```python
from build123d import *

# Parameters (mm, degrees)
BOSS_EXTRUDE1_DEPTH             = 1.5
BOSS_EXTRUDE2_DEPTH             = 1.5
BOSS_EXTRUDE3_DEPTH             = 1.5
CUT_EXTRUDE1_START              = -4
SKETCH2_R                       = 2.25
CUT_EXTRUDE1_DEPTH              = 5
CIRPATTERN1_COUNT               = 3
CIRPATTERN1_ANGLE               = 60
CIRPATTERN1_THE_OTHER_WAY_COUNT = 3
CIRPATTERN1_THE_OTHER_WAY_ANGLE = 60
CUT_EXTRUDE2_START              = -4
SKETCH6_R                       = 3.25
CUT_EXTRUDE2_DEPTH              = 5
LPATTERN1_COUNT                 = 3
LPATTERN1_PITCH                 = 12.5
SKETCH7_R                       = 3.25
CUT_EXTRUDE3_DEPTH              = 10
LPATTERN2_COUNT                 = 4
LPATTERN2_PITCH                 = 12


with BuildPart() as part:
    # Sketch1 → Boss-Extrude1 (new body, symmetric)
    with BuildSketch(Plane(origin=(0, 0, 0), x_dir=(1, 0, 0), z_dir=(0, 1, 0))):
        with BuildLine():
            Line((0, 33), (0, 43))
            ThreePointArc((0, 43), (41.53481053, 11.129218939), (21.5, -37.239092363))
            Line((21.5, -37.239092363), (16.5, -28.578838325))
            ThreePointArc((16.5, -28.578838325), (31.875552268, 8.541028488), (0, 33))
        make_face()
    extrude(amount=BOSS_EXTRUDE1_DEPTH, both=True)

    # Sketch4 → Boss-Extrude2 (add, symmetric)
    with BuildSketch(Plane(origin=(0, 0, 0), x_dir=(1, 0, 0), z_dir=(0, 1, 0))):
        Polygon((90.122106501, 50.030050167), (25.40507614, 32.689174146), (38.346028395, -15.607117169), (103.063058756, 1.733758853), align=None)
    extrude(amount=BOSS_EXTRUDE2_DEPTH, both=True)

    # Sketch5 → Boss-Extrude3 (add, symmetric)
    with BuildSketch(Plane(origin=(0, 0, 0), x_dir=(1, 0, 0), z_dir=(0, 1, 0))):
        Polygon((0, 43), (58.722616268, 41.616582117), (27.323126035, 33.203114066), align=None)
        Polygon((71.663568523, -6.679709198), (40.26407829, -15.093177248), (21.5, -37.239092363), align=None)
    extrude(amount=BOSS_EXTRUDE3_DEPTH, both=True)

    # Sketch2 → Cut-Extrude1 (cut)
    with BuildSketch(Plane(origin=(0, 1.5, 0), x_dir=(1, 0, 0), z_dir=(0, 1, 0)).offset(CUT_EXTRUDE1_START)):
        with Locations((36.757261811, 9.638656763)):
            Circle(SKETCH2_R)
    cut_extrude1 = extrude(amount=CUT_EXTRUDE1_DEPTH, mode=Mode.SUBTRACT)

    # CirPattern1: Cut-Extrude1 ×3 about axis
    cirpattern1_axis = Axis((0, 0, 0), (0, -1, 0))
    for i in range(1, CIRPATTERN1_COUNT):
        add(cut_extrude1.rotate(cirpattern1_axis, i * CIRPATTERN1_ANGLE / (CIRPATTERN1_COUNT - 1)), mode=Mode.SUBTRACT)

    # CirPattern1 the other way: Cut-Extrude1 ×3 about axis
    cirpattern1_the_other_way_axis = Axis((0, 0, 0), (0, 1, 0))
    for i in range(1, CIRPATTERN1_THE_OTHER_WAY_COUNT):
        add(cut_extrude1.rotate(cirpattern1_the_other_way_axis, i * CIRPATTERN1_THE_OTHER_WAY_ANGLE / (CIRPATTERN1_THE_OTHER_WAY_COUNT - 1)), mode=Mode.SUBTRACT)

    # Sketch6 → Cut-Extrude2 (cut)
    with BuildSketch(Plane(origin=(0, 1.5, 0), x_dir=(1, 0, 0), z_dir=(0, 1, 0)).offset(CUT_EXTRUDE2_START)):
        with Locations((94.679313348, 9.840102845)):
            Circle(SKETCH6_R)
        with Locations((86.914741995, 38.817877634)):
            Circle(SKETCH6_R)
    cut_extrude2 = extrude(amount=CUT_EXTRUDE2_DEPTH, mode=Mode.SUBTRACT)

    # LPattern1: Cut-Extrude2 ×3
    with Locations(*[Vector(-0.965925826, 0, 0.258819045) * (i * LPATTERN1_PITCH) for i in range(1, LPATTERN1_COUNT)]):
        add(cut_extrude2, mode=Mode.SUBTRACT)

    # Sketch7 → Cut-Extrude3 (cut)
    with BuildSketch(Plane(origin=(0, 1.5, 0), x_dir=(1, 0, 0), z_dir=(0, 1, 0))):
        with Locations((90.797027671, 24.32899024)):
            Circle(SKETCH7_R)
    cut_extrude3 = extrude(amount=-CUT_EXTRUDE3_DEPTH, mode=Mode.SUBTRACT)

    # LPattern2: Cut-Extrude3 ×4
    with Locations(*[Vector(-0.965925826, 0, 0.258819045) * (i * LPATTERN2_PITCH) for i in range(1, LPATTERN2_COUNT)]):
        add(cut_extrude3, mode=Mode.SUBTRACT)


solid = part.part
```
CAD build for the part. Positions are in the model's coordinates, mm. Give positions to 0.01 mm unless a question says otherwise; leave off trailing zeros. Write each loop counter-clockwise with the first axis right and the second up, starting at its lowest first coordinate (ties: lowest second). Pieces come first, ordered by that corner, then holes. Notation, with made-up numbers: M 12.5,17.25 L 16.5,17.25 A32 ccw 16.5,47.25 Z; hole C 8,80 d11. An arc over 180 degrees is marked long. Return JSON: item names as keys, results as strings. Group by question number.
(1) Drill centre lines: L1, parallel to Z at x = 36, y = 1.1; L2, parallel to Z at x = 38, y = 0.4; L3, parallel to X at y = 1.2, z = -22.5. Where is each one in solid material? Low to high. Write a range as [from, to].
(2) Band-saw the part on A-A (x = 31.5). Give the cut face in (y, z), and give its area (3 significant figures).
(3) Flat gauge pin, fed straight in: pin 1 Ø1 at (x, y) = (40, 1) entering from -Z. Where does the tip first touch, or does it go through?
(4) Band-saw the part on B-B (y = 0.65). State how many separate pieces and enclosed holes the cut face has, and give its area (3 significant figures).
(5) Band-saw the part on D-D (z = 20.5). Give the cut face in (x, y), and give its area (3 significant figures).
(6) Band-saw the part on C-C (x = 61). Give the cut face in (y, z).
(7) Mould opens along X. For faces 1 (the face through (28.384, -0.021, 28.534)), 2 (the face through (51, -1.5, -17)), 3 (the face through (96.683, 0.021, -25.544)) say: pulls with the +X half, pulls with the -X half, needs draft (parallel to the pull), parting line crosses it, or undercut.
Entries:
{
 "1": {"L1": "z = [-42.15, -11.76], [-7.52, 7.88], [12.18, 28.41]", "L2": "z = [-42.1, -11.51], [-7.76, 8.23], [11.83, 27.19]", "L3": "x = [24.14, 76.22], [82.19, 88.11], [93.48, 97.5]"},
 "2": {"outline": "M -1.5,-42.26 L 1.5,-42.26 L 1.5,-9.84 L -1.5,-9.84 Z; M -1.5,9.84 L 1.5,9.84 L 1.5,31.15 L -1.5,31.15 Z", "area": "161 mm^2"},
 "3": {"pin 1": "stops at z = -42.07"},
 "4": {"separate pieces": "1", "enclosed holes": "15", "area": "4,000 mm^2"},
 "5": {"outline": "M 25.86,-1.5 L 48.98,-1.5 L 48.98,1.5 L 25.86,1.5 Z", "area": "69.4 mm^2"},
 "6": {"outline": "M -1.5,-42.23 L 1.5,-42.23 L 1.5,-35.08 L -1.5,-35.08 Z; M -1.5,-29.62 L 1.5,-29.62 L 1.5,13.18 L -1.5,13.18 Z"},
 "7": {"face 1": "undercut", "face 2": "needs draft", "face 3": "pulls with the +X half"}
}
